Can you work these out from the drawing? Everything is in mm from the part's minimum corner. Round coordinates to 2 decimals unless told otherwise and drop trailing zeros. Loops run counter-clockwise (first coordinate to the right, second up) from the corner with the lowest first, then second, coordinate; pieces in that order, holes last. Notation, with made-up numbers: (21.25, 65) -> (29.25, 65) arc R19 ccw to (29.25, 76) -> close; hole circle Ø7 at (-19, -5). An arc over 180 degrees is marked (long way). Answer as a JSON object with one key per item and string values.
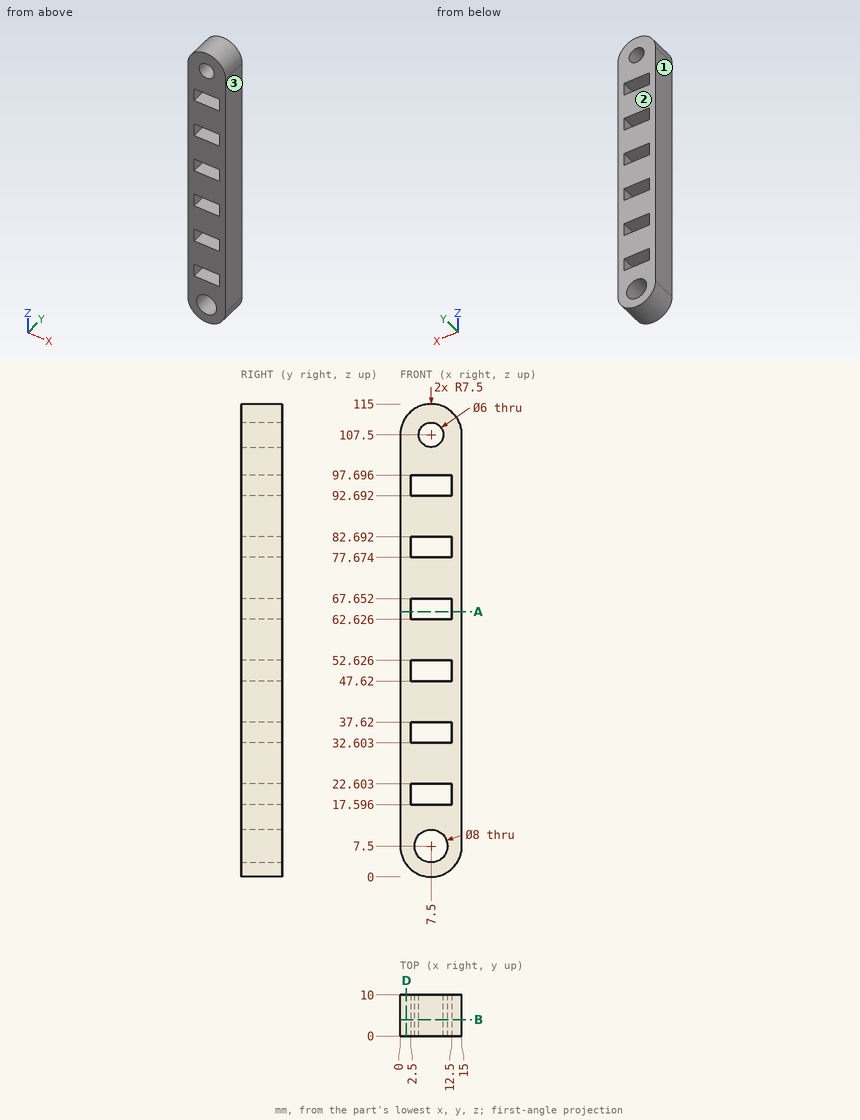
Q1. I'm going to push flat-ended pins straight in: pin 1 (5.5 mm diameter, centred on y = 6, z = 34, fed in from -X); pin 2 (4 mm diameter, centred on x = 11.5, y = 6.5, fed in from +Z); pin 3 (4 mm diameter, centred on x = 13, y = 7, fed in from +Z); pin 4 (3 mm diameter, centred on x = 1.5, y = 5, fed in from -Z). Where does each tip first touch, or does it pass through?
Determined:
{"pin 1": "x = 0", "pin 2": "z = 114.73", "pin 3": "z = 114.13", "pin 4": "z = 1.5"}
Q2. I want a section at B-B, the plane y = 4. Give the number of separate pieces and of enclosed holes in the cut face, then the cut area to 3 significant figures.
Determined:
{"separate pieces": "1", "enclosed holes": "8", "area": "1,300 mm²"}
Q3. I want a section at A-A, the plane z = 64.5. Write out the boundary of the cut face in (x, y), then the cut area to 3 significant figures.
Determined:
{"outline": "(0, 0) -> (2.5, 0) -> (2.5, 10) -> (0, 10) -> close; (12.5, 0) -> (15, 0) -> (15, 10) -> (12.5, 10) -> close", "area": "50.0 mm²"}
Q4. If I drill on L1, parallel to X at y = 4.75, z = 107.5; L2, parallel to X at y = 1.5, z = 95, over which ranges is the centre line in solid material (lowest first)? Write a range as [from, to].
Determined:
{"L1": "[0, 4.5], [10.5, 15]", "L2": "[0, 2.5], [12.5, 15]"}
Q5. We'd pull the mould along X, two halves only. Please class the marked faces 1, 2 and 3: pulls with the +X half, pulls with the -X half, needs draft (parallel to the pull), parting line crosses it, or undercut.
Determined:
{"face 1": "pulls with the -X half", "face 2": "needs draft", "face 3": "pulls with the +X half"}
Q6. I want a section at D-D, the plane x = 1.5. Write out the boundary of the cut face in (y, z).
Determined:
{"outline": "(0, 3) -> (10, 3) -> (10, 112) -> (0, 112) -> close"}
